Geometry check sheet. Reference: the model listing, model coordinates, mm. A direction names the side the tool comes from. Round coordinates to 2 decimals unless told otherwise and drop trailing zeros. Write each loop counter-clockwise with the first axis right and the second up, starting at its lowest first coordinate (ties: lowest second). Pieces come first, ordered by that corner, then holes. Notation, with made-up numbers: M 41.5,77.25 L 69.5,77.25 A13 ccw 69.5,93.25 Z; hole C 33.5,3 d8. An arc over 180 degrees is marked long. One line per item, written item: value. Start each with the question number.
1. Access from +Z, -Z, +X, -X, +Y, -Y to the whole of each face (thin tool, end or side, straight path). Record for faces 1 (the flat face through (4.2, 0, 0.1)), 2 (the cylindrical face through (-3.905, 2.958, -0.867)).
2. Section check C-C (z = 5.5). Record the boundary of the cut face in (x, y).
3. Depth check by flat-ended pin: P1, Ø2, axis at x = 2, y = -1.5, coming from the +Z side; P2, Ø2, axis at y = -0.5, z = -8, coming from the -X side; P3, Ø5, axis at x = -3.5, z = -2.5, coming from the -Y side; P4, Ø4, axis at y = 3, z = -2, coming from the -X side. Enter the tip coordinate at first touch or a pass-through.
4. Scan lines: probe 1 along X at (y, z) = (3.4, 0); probe 2 along Y at (x, z) = (3.5, 3.25); probe 3 along Z at (x, y) = (5, -0.5). Record each from-to range of solid material in increasing order. Write a range as [from, to].
5. Section check D-D (x = 8.5). Record the boundary of the cut face in (y, z).
6. Section check B-B (y = 3). Record the boundary of the cut face in (x, z).
7. Release check for a two-part mould opening along X. For faces 3 (the cylindrical face through (3.755, 1.944, 11.923)), 4 (the flat face through (3, 6, -3)), 5 (the flat face through (0, -1, 8.538)) record: pulls with the +X half, pulls with the -X half, needs draft (parallel to the pull), parting line crosses it, or undercut.
8. Section check A-A (x = 0). Record the boundary of the cut face in (y, z), and give its area (3 significant figures).
from build123d import *

# Parameters (mm, degrees)
BOSS_EXTRUDE1_DEPTH      = 6
BOSS_EXTRUDE1_DEPTH_BACK = 2
SKETCH1_R                = 12.5
SKETCH1_R_2              = 4
CUT_EXTRUDE1_DEPTH       = 2


with BuildPart() as part:
    # Sketch1 → Boss-Extrude1 (new, two sides: drawn at the far end of the back side and taken through both)
    with BuildSketch(Plane(origin=(0, 0, 0), x_dir=(1, 0, 0), z_dir=(0, 1, 0)).offset(-BOSS_EXTRUDE1_DEPTH_BACK)):
        with Locations(Location((0, 0, 0), (0, 0, 270))):
            Circle(SKETCH1_R)
        with Locations(Location((0, 0, 0), (0, 0, 270))):
            Circle(SKETCH1_R_2, mode=Mode.SUBTRACT)
    extrude(amount=BOSS_EXTRUDE1_DEPTH + BOSS_EXTRUDE1_DEPTH_BACK)

    # Sketch2 → Cut-Extrude1 (cut)
    with BuildSketch(Plane.XZ.offset(2)):
        Polygon((9.85829335, 0), (4.929146675, 8.537532479), (-4.929146675, 8.537532479), (-9.85829335, 0), (-4.929146675, -8.537532479), (4.929146675, -8.537532479), align=None)
    extrude(amount=-CUT_EXTRUDE1_DEPTH, mode=Mode.SUBTRACT)


solid = part.part
Result sheet:
1. face 1: -Y
1. face 2: +Y, -Y
2. outline: M -11.22,-2 L -6.68,-2 L -6.68,0 L 6.68,0 L 6.68,-2 L 11.22,-2 L 11.22,6 L -11.22,6 Z
3. P1: stops at z = 12.46
3. P2: stops at x = -10.36
3. P3: stops at y = 0
3. P4: stops at x = -12.5
4. probe 1: x = [-12.5, -4], [4, 12.5]
4. probe 2: y = [0, 6]
4. probe 3: z = [-11.46, -8.41], [8.41, 11.46]
5. outline: M -2,-9.17 L 6,-9.17 L 6,9.17 L -2,9.17 L -2,2.35 L 0,2.35 L 0,-2.35 L -2,-2.35 Z
6. outline: C 0,0 d25; hole C 0,0 d8
7. face 3: parting line crosses it
7. face 4: needs draft
7. face 5: undercut
8. outline: M -2,-12.5 L 6,-12.5 L 6,-4 L 0,-4 L 0,-8.54 L -2,-8.54 Z; M -2,8.54 L 0,8.54 L 0,4 L 6,4 L 6,12.5 L -2,12.5 Z
8. area: 118 mm2
